The model under review builds one solid part; all positions refer to its coordinate system, in mm. A direction names the side the tool comes from. Round coordinates to 2 decimals unless told otherwise and drop trailing zeros. Order: outer loops, then holes, each group sorted by start corner. A loop starts at its lowest first (then second) coordinate and runs counter-clockwise, first axis right, second up.
1) Consider section A-A (y = 0). Give the boundary of the cut face in (x, z) (3 decimals).
2) To check wall thickness, follow L1, parallel to X at y = 32, z = 47.5; L2, parallel to X at y = -17, z = 48; L3, parallel to Y at x = 33.5, z = 36. State the ranges of each line that lie inside material, in increasing order.
3) Clearance check with flat-ended pins moving along their axes: P1, Ø6, axis at y = -22, z = 29, coming from the +X side; P2, Ø3, axis at x = -10, z = 10, coming from the +Y side; P3, Ø4, axis at x = 26.5, z = 34.5, coming from the -Y side; P4, Ø5, axis at x = 0, y = 0, coming from the +Z side. State where each tip first meets the part, or that it passes through.
4) Mouldability with a two-part tool opening along X and no side actions: class faces 4 (the face through (-25, 22, 50.8)), 5 (the face through (34.333, 11.131, 37.922)) as pulls with the +X half, pulls with the -X half, needs draft (parallel to the pull), parting line crosses it, or undercut.
5) Consider section D-D (z = 5). Give the boundary of the cut face in (x, y) (3 decimals).
6) Consider section C-C (x = 0). Give the boundary of the cut face in (y, z) (3 decimals), then the cut area to 3 significant figures.
7) Consider section B-B (z = 32). Give the number of separate pieces and of enclosed holes in the cut face, then the cut area to 3 significant figures.
8) Machinability: for faces 1 (the face through (-8.4, -26.68, 12.57)), 2 (the face through (20, -27, 50.8)), 3 (the face through (24.6, 24.97, 37.92)), which of the approach directions +Z, -Z, +X, -X, +Y, -Y give a long, thin tool a straight path to every point of the face, cutting with its end or side? Answer none if there is none.
from build123d import *

# Parameters (mm, degrees)
F0_R     = 38.1
F0_R_2   = 3.175
F1_DEPTH = 25.4
F2_R     = 2.54
F3_DEPTH = 25.4


with BuildPart() as f1:
    # F0 (on Top) → F1 (new body)
    with BuildSketch(Plane.XY):
        Circle(F0_R)
        Circle(F0_R_2, mode=Mode.SUBTRACT)
    extrude(amount=F1_DEPTH)

    # F2 (on face) → F3 (join)
    with BuildSketch(Plane.XY.offset(25.4)):
        with Locations((13.647064, 30.651807)):
            Circle(F2_R)
        with Locations((0, 33.55258)):
            Circle(F2_R)
        with Locations((-13.647064, 30.651807)):
            Circle(F2_R)
        with Locations((-24.934426, 22.451058)):
            Circle(F2_R)
        with Locations((-31.910399, 10.368317)):
            Circle(F2_R)
        with Locations((-33.368775, -3.5072)):
            Circle(F2_R)
        with Locations((-29.057386, -16.77629)):
            Circle(F2_R)
        with Locations((-19.721711, -27.144607)):
            Circle(F2_R)
        with Locations((-6.975974, -32.819375)):
            Circle(F2_R)
        with Locations((6.975974, -32.819375)):
            Circle(F2_R)
        with Locations((19.721711, -27.144607)):
            Circle(F2_R)
        with Locations((29.057386, -16.77629)):
            Circle(F2_R)
        with Locations((33.368775, -3.5072)):
            Circle(F2_R)
        with Locations((31.910399, 10.368317)):
            Circle(F2_R)
        with Locations((24.934426, 22.451058)):
            Circle(F2_R)
    extrude(amount=F3_DEPTH)

    # F5 (on Right) → F6 (revolve, cut)
    with BuildSketch(Plane.YZ):
        Polygon((-27.45885, 12.864876), (-38.457373, 19.214876), (-38.457373, 6.514876), align=None)
    revolve(axis=Axis((0, 0, 4.729655), (0, 0, -1)), mode=Mode.SUBTRACT)


solid = f1.part
Answer below:
1. outline: (-38.1, 0) - (-3.175, 0) - (-3.175, 25.4) - (-38.1, 25.4) - (-38.1, 19.009) - (-27.459, 12.865) - (-38.1, 6.721) - close; (3.175, 0) - (38.1, 0) - (38.1, 6.721) - (27.459, 12.865) - (38.1, 19.009) - (38.1, 25.4) - (3.175, 25.4) - close
2. L1: x = -15.8 to -11.49, -2.01 to 2.01, 11.49 to 15.8
2. L2: x = -31.59 to -26.53, 26.53 to 31.59
2. L3: y = -6.04 to -0.97, 8.39 to 12.35
3. P1: stops at x = 30.28
3. P2: stops at y = 33.6
3. P3: stops at y = -19.25
3. P4: passes through
4. face 4: needs draft
4. face 5: undercut
5. outline: circle Ø76.2 at (0, 0); hole circle Ø6.35 at (0, 0)
6. outline: (-38.1, 0) - (-3.175, 0) - (-3.175, 25.4) - (-38.1, 25.4) - (-38.1, 19.009) - (-27.459, 12.865) - (-38.1, 6.721) - close; (3.175, 0) - (38.1, 0) - (38.1, 6.721) - (27.459, 12.865) - (38.1, 19.009) - (38.1, 25.4) - (36.093, 25.4) - (36.093, 50.8) - (31.013, 50.8) - (31.013, 25.4) - (3.175, 25.4) - close
6. area: 1,770 mm2
7. separate pieces: 15
7. enclosed holes: 0
7. area: 304 mm2
8. face 1: none
8. face 2: +Z, +X, -X, +Y, -Y
8. face 3: +Z
